Input: part model. Units: mm. Frame: model coordinates. A direction names the side the tool comes from. Coordinates: 2 decimals unless noted, no trailing zeros. Order: outer loops, then holes, each group sorted by start corner. A loop starts at its lowest first (then second) coordinate and runs counter-clockwise, first axis right, second up. Notation, with made-up numbers: M 8.25,77.5 L 37.25,77.5 A28 ccw 37.25,110.5 Z; hole C 23,72.25 d4. An arc over 180 degrees is marked long. One line per item, written item: value.
```python
from build123d import *

# Parameters (mm, degrees)
F3_DEPTH = 31.75
F5_DEPTH = 4.48238
F6_R     = 5.08


with BuildPart() as f3:
    # F2 (on Front) → F3 (new body)
    with BuildSketch(Plane.XZ):
        Polygon((444.5, 0), (444.5, 4.48138), (355.574593, 3.902439), (355.6, 0), align=None)
    extrude(amount=F3_DEPTH)

    # F4 (on face) → F5 (cut, through all)
    with BuildSketch(Plane(origin=(0, 0, 0), x_dir=(1, 0, 0), z_dir=(0, 0, -1))):
        with BuildLine():
            Line((434.975, 25.4), (365.099593, 25.4))
            ThreePointArc((365.099593, 25.4), (362.854529, 24.470064), (361.924593, 22.225))
            Line((361.924593, 22.225), (361.924593, 9.525))
            ThreePointArc((361.924593, 9.525), (362.854529, 7.279936), (365.099593, 6.35))
            Line((365.099593, 6.35), (434.975, 6.35))
            ThreePointArc((434.975, 6.35), (437.220064, 7.279936), (438.15, 9.525))
            Line((438.15, 9.525), (438.15, 22.225))
            ThreePointArc((438.15, 22.225), (437.220064, 24.470064), (434.975, 25.4))
        make_face()
    extrude(amount=-F5_DEPTH, mode=Mode.SUBTRACT)

    # F6
    f6_edges = [f3.edges().sort_by_distance(p)[0] for p in [
        (444.5, -31.75, 2.24069),
        (355.587297, -31.75, 1.951219),
        (355.587297, 0, 1.951219),
        (444.5, 0, 2.24069),
    ]]
    fillet(f6_edges, radius=F6_R)


solid = f3.part
```
(1) Cut plane B-B on y = -17.5. Output: boundary loops of the cut face in (x, z).
Data:
outline: M 355.57,3.9 L 355.6,0 L 361.92,0 L 361.92,3.94 Z; M 438.15,0 L 444.5,0 L 444.5,4.48 L 438.15,4.44 Z
(2) Draft query along Y for faces 1 (the flat face through (444.5, -16, 2)), 2 (the flat face through (361.925, -16, 2)), 3 (the cylindrical face through (357.115, -1.449, 1.917)), 4 (the cylindrical face through (362.83, -7.305, 1.954)). Return one class per face: released by +Y, released by -Y, zero draft, split by the parting line, or undercut.
Data:
face 1: zero draft
face 2: undercut
face 3: released by +Y
face 4: undercut
(3) First-contact query: pin 1 (2 mm diameter, centred on y = -16.5, z = 2, fed in from -X). Flat tip, straight axial feed; report the tip coordinate or a pass-through.
Data:
pin 1: stops at x = 355.58
(4) Access query for faces 5 (the flat face through (401, -25.4, 2)), 6 (the cylindrical face through (443.051, -30.222, 2.272)). Directions: +Z, -Z, +X, -X, +Y, -Y. A direction counts if a zero-diameter tool reaches every point of the face in a straight line with its end or side. Return the directions, or none.
Data:
face 5: +Z, -Z
face 6: +Z, -Z, +X, -Y
(5) Cut plane A-A on x = 408. Output: boundary loops of the cut face in (y, z).
Data:
outline: M -31.75,0 L -25.4,0 L -25.4,4.24 L -31.75,4.24 Z; M -6.35,0 L 0,0 L 0,4.24 L -6.35,4.24 Z
(6) Ray query, line 1 (Y direction, x = 385, z = 3.2); line 2 (X direction, y = -14.5, z = 2.35); line 3 (Y direction, x = 362.5, z = 2.6). Return the intervals inside material, ascending. Write a range as from..to.
Data:
line 1: y = -31.75..-25.4, -6.35..0
line 2: x = 355.58..361.92, 438.15..444.5
line 3: y = -31.75..-24.05, -7.7..0
(7) Cut plane C-C on y = -29. Output: boundary loops of the cut face in (x, z), plus the area to 3 significant figures.
Data:
outline: M 356.14,3.91 L 356.17,0 L 443.93,0 L 443.93,4.48 Z
area: 368 mm2
